Geometry check sheet. Reference: the model listing, model coordinates, mm. A direction names the side the tool comes from. Coordinates: 2 decimals unless noted, no trailing zeros. Order: outer loops, then holes, each group sorted by start corner. A loop starts at its lowest first (then second) coordinate and runs counter-clockwise, first axis right, second up. Notation, with made-up numbers: M -25,-22.75 L 15,-22.75 A11 ccw 15,-16.75 Z; hole C -40,28.25 d11. An arc over 180 degrees is marked long. One line per item, written item: value. Start each with the question number.
1) Go/stop test with flat-tipped pins: P1, Ø3.5, axis at x = 15, y = 34, coming from the -Z side; P2, Ø8, axis at x = 12, z = -19.5, coming from the +Y side. Record where each tip stops, or that it passes through.
2) Sectioned sample at A-A, the plane z = -33. Enter the section's corners in (x, y), then the cut area to 3 significant figures.
3) Sectioned sample at D-D, the plane y = 34. Enter the section's corners in (x, z).
4) Access from +Z, -Z, +X, -X, +Y, -Y to the whole of each face (thin tool, end or side, straight path). Record for faces 4 (the flat face through (10, 21, -54)), 5 (the cylindrical face through (10, 39, -55)).
5) Sectioned sample at B-B, the plane x = 10. Enter the section's corners in (y, z).
6) Sectioned sample at C-C, the plane y = 21.5. Enter the section's corners in (x, z).
7) Thickness scan on L1, parallel to X at y = 24, z = -1; L2, parallel to Z at x = 1.75, y = 18; L3, parallel to Y at x = 5, z = -55.5. Record the ranges inside material, lowest first. Write a range as from..to.
8) Draft check along X on faces 1 (the cylindrical face through (10, 39, -1)), 2 (the flat face through (5, 2, -28)), 3 (the cylindrical face through (13.92, 35.18, -55.01)). Enter one of: pulls with the +X half, pulls with the -X half, needs draft (parallel to the pull), parting line crosses it, or undercut.
Autodesk Inventor part; units mm, degrees
ref_plane "YZ Plane" through (0, 0, 0) normal (1, 0, 0) x (0, 1, 0)
ref_plane "XZ Plane" through (0, 0, 0) normal (0, 1, 0) x (-1, 0, 0)
ref_plane "XY Plane" through (0, 0, 0) normal (0, 0, 1) x (1, 0, 0)
sketch "スケッチ1" plane through (0, 0, 0) normal (1, 0, 0) x (0, 1, 0)
  line L0 (0, 0) -> (2, 0)
  line L1 (2, 0) -> (2, -56)
  line L2 (2, -56) -> (0, -56)
  line L3 (0, -56) -> (0, 0)
  line L4 (2, 0) -> (39, 0)
  line L5 (39, 0) -> (39, -2)
  line L6 (39, -2) -> (2, -2)
  line L7 (2, -2) -> (2, 0)
  line L8 (2, -56) -> (39, -56)
  line L9 (39, -56) -> (39, -54)
  line L10 (39, -54) -> (2, -54)
  line L11 (2, -54) -> (2, -56)
  point P0 (2, -54)
  point P1 (2, -2)
  dimension "d0" = 2
  dimension "d1" = 56
  dimension "d2" = 37
  dimension "d3" = 2
  dimension "d4" = 37
  dimension "d5" = 2
extrude "押し出し1" add sketch "スケッチ1" along normal blind 20
sketch "スケッチ2" plane through (0, 0, 0) normal (0, 0, 1) x (1, 0, 0)
  arc A0 (20, 29) -> (0, 29) centre (10, 29) ccw
  line L0 (0, 39) -> (20, 39)
  line L1 (0, 39) -> (0, 0)
  line L2 (20, 39) -> (20, 0)
  point P0 (10, 39)
  dimension "d8" = 10
extrude "押し出し2" cut sketch "スケッチ2" against normal through all
sketch "スケッチ3" plane through (0, 0, 0) normal (0, 0, 1) x (1, 0, 0)
  arc A0 (20, 29) -> (0, 29) centre (10, 29) ccw
  point P0 (0, 0)
  point P1 (5, 34)
  point P2 (15, 34)
  point P3 (15, 24)
  point P4 (5, 24)
  dimension "d11" = 5
  dimension "d12" = 5
  dimension "d13" = 10
  dimension "d14" = 10
hole "穴1" at (5, 34, 0) at (15, 34, 0) at (15, 24, 0) at (5, 24, 0) direction (0, 0, -1) diameter 3.2 end through all
sketch "スケッチ4" plane through (0, 0, 0) normal (0, 0, 1) x (1, 0, 0)
  arc A0 (20, 29) -> (0, 29) centre (10, 29) ccw
  circle A1 centre (10, 29) radius 4
  point P0 (0, 0)
  dimension "d22" = 8
extrude "押し出し3" cut sketch "スケッチ4" against normal through all
fillet "フィレット1" radius 0.5 2 edges at (10, 2, -54) (10, 2, -2)
fillet "フィレット2" radius 2 2 edges at (10, 0, -56) (10, 0, 0)
sketch "スケッチ5" plane through (0, 2, -2.5) normal (0, 1, 0) x (1, 0, 0)
  line L0 (0, -0.5) -> (0, 51.5)
  line L1 (0, 25.5) -> (20, 25.5)
  line L2 (20, 51) -> (20, 0)
  line L3 (20, 51.5) -> (0, 51.5)
  line L4 (10, 51.5) -> (10, 0)
  line L5 (20, 0) -> (0, 0)
  point P0 (0, -2.5)
  point P1 (5, 30.5)
  point P2 (15, 30.5)
  point P3 (15, 20.5)
  point P4 (5, 20.5)
  dimension "d27" = 10
  dimension "d28" = 10
hole "穴2" at (5, 2, -33) at (15, 2, -33) at (15, 2, -23) at (5, 2, -23) direction (0, -1, 0) diameter 3.2 end through all
sketch "スケッチ6" plane through (0, 2, -2.5) normal (0, 1, 0) x (1, 0, 0)
  circle A0 centre (10, 25.5) radius 3
  circle A1 centre (5, 20.5) radius 1.6
  point P0 (0, -2.5)
  dimension "d36" = 6
  dimension "d37" = 5
  dimension "d38" = 5
extrude "押し出し4" cut sketch "スケッチ6" against normal through all contours A0
properties part number "サーボモーター25kgcmサーボホーン2" material "アルミニウム 6061"
Final values:
1. P1: stops at z = -56
1. P2: stops at y = 2
2. outline: M 0,0 L 3.4,0 L 3.4,2 L 0,2 Z; M 6.6,0 L 13.4,0 L 13.4,2 L 6.6,2 Z; M 16.6,0 L 20,0 L 20,2 L 16.6,2 Z
2. area: 27.2 mm^2
3. outline: M 1.34,-56 L 3.4,-56 L 3.4,-54 L 1.34,-54 Z; M 1.34,-2 L 3.4,-2 L 3.4,0 L 1.34,0 Z; M 6.6,-56 L 13.4,-56 L 13.4,-54 L 6.6,-54 Z; M 6.6,-2 L 13.4,-2 L 13.4,0 L 6.6,0 Z; M 16.6,-56 L 18.66,-56 L 18.66,-54 L 16.6,-54 Z; M 16.6,-2 L 18.66,-2 L 18.66,0 L 16.6,0 Z
4. face 4: +X, -X, +Y
4. face 5: +Z, -Z, +Y
5. outline: M 0,-54 A2 ccw 2,-56 L 25,-56 L 25,-54 L 2.5,-54 A0.5 cw 2,-53.5 L 2,-31 L 0,-31 Z; M 0,-25 L 2,-25 L 2,-2.5 A0.5 cw 2.5,-2 L 25,-2 L 25,0 L 2,0 A2 ccw 0,-2 Z; M 33,-56 L 39,-56 L 39,-54 L 33,-54 Z; M 33,-2 L 39,-2 L 39,0 L 33,0 Z
6. outline: M 0,-56 L 20,-56 L 20,-54 L 0,-54 Z; M 0,-2 L 20,-2 L 20,0 L 0,0 Z
7. L1: x = 0..3.4, 6.6..13.4, 16.6..20
7. L2: z = -56..-54, -2..0
7. L3: y = 0.68..22.4, 25.6..32.4, 35.6..37.66
8. face 1: parting line crosses it
8. face 2: needs draft
8. face 3: undercut
